Could you check a few things on this model? Use its own coordinates, in mm. A direction names the side the tool comes from. Round coordinates to 2 decimals unless told otherwise and drop trailing zeros. Loops run counter-clockwise (first coordinate to the right, second up) from the corner with the lowest first, then second, coordinate; pieces in that order, holes last. Notation, with made-up numbers: M -26.5,24 L -7.5,24 A22 cw -7.5,48 Z; hole C -10,76.5 d7. An arc over 180 degrees is marked long. Answer in a Markdown table with one row per item.
```python
from build123d import *

# Parameters (mm, degrees)
F1_DEPTH = 436.5625
F2_R     = 5.55625
F3_DEPTH = 50.801
F4_R     = 5.55625
F5_DEPTH = 50.801


with BuildPart() as f1:
    # F0 (on Right) → F1 (new body)
    with BuildSketch(Plane.YZ):
        Polygon((0, 50.8), (0, 0), (50.8, 0), (50.8, 6.35), (6.35, 6.35), (6.35, 50.8), align=None)
    extrude(amount=F1_DEPTH)

    # F2 (on face) → F3 (cut, through all)
    with BuildSketch(Plane.XZ):
        with Locations((25.4, 25.4)):
            Circle(F2_R)
        with BuildLine():
            ThreePointArc((144.4625, 30.1625), (139.7, 25.4), (144.4625, 20.6375))
            Line((144.4625, 20.6375), (160.3375, 20.6375))
            ThreePointArc((160.3375, 20.6375), (165.1, 25.4), (160.3375, 30.1625))
            Line((160.3375, 30.1625), (144.4625, 30.1625))
        make_face()
        with BuildLine():
            ThreePointArc((400.84375, 30.1625), (396.08125, 25.4), (400.84375, 20.6375))
            Line((400.84375, 20.6375), (416.71875, 20.6375))
            ThreePointArc((416.71875, 20.6375), (421.48125, 25.4), (416.71875, 30.1625))
            Line((416.71875, 30.1625), (400.84375, 30.1625))
        make_face()
    extrude(amount=-F3_DEPTH, mode=Mode.SUBTRACT)

    # F4 (on face) → F5 (cut, through all)
    with BuildSketch(Plane(origin=(0, 0, 0), x_dir=(1, 0, 0), z_dir=(0, 0, -1))):
        with Locations((227.80625, -25.4)):
            Circle(F4_R)
        with Locations((177.00625, -25.4)):
            Circle(F4_R)
    extrude(amount=-F5_DEPTH, mode=Mode.SUBTRACT)


solid = f1.part
```
1) I want a section at A-A, the plane y = 25.4. Please give me the cut outline in (x, z), plus the area to 3 significant figures.
Computed:
| item | result |
|---|---|
| outline | M 0,0 L 171.45,0 L 171.45,6.35 L 0,6.35 Z; M 182.56,0 L 222.25,0 L 222.25,6.35 L 182.56,6.35 Z; M 233.36,0 L 436.56,0 L 436.56,6.35 L 233.36,6.35 Z |
| area | 2,630 mm² |
2) I want a section at C-C, the plane x = 25.4. Please give me the cut outline in (y, z).
Computed:
| item | result |
|---|---|
| outline | M 0,0 L 50.8,0 L 50.8,6.35 L 6.35,6.35 L 6.35,19.84 L 0,19.84 Z; M 0,30.96 L 6.35,30.96 L 6.35,50.8 L 0,50.8 Z |
3) Which directions (+Z, -Z, +X, -X, +Y, -Y) give clear straight access to the entire face, cutting with the end or side of a thin tool? Please do faces 1 (the face through (215, 6.35, 28)), 2 (the face through (436.562, 14, 5)).
Computed:
| item | result |
|---|---|
| face 1 | +Z, +X, -X, +Y |
| face 2 | +Z, -Z, +X, +Y, -Y |
4) I want a section at D-D, the plane y = 46. Please give me the cut outline in (x, z), plus the area to 3 significant figures.
Computed:
| item | result |
|---|---|
| outline | M 0,0 L 436.56,0 L 436.56,6.35 L 0,6.35 Z |
| area | 2,770 mm² |
5) I need wall thicknesses on line 1 (X direction, y = 25.4, z = 4.5); line 2 (Z direction, x = 25.4, y = 3.5); line 3 (X direction, y = 1, z = 25). Which ranges of each line are inside material? Lowest first, please.
Computed:
| item | result |
|---|---|
| line 1 | x = 0 to 171.45, 182.56 to 222.25, 233.36 to 436.56 |
| line 2 | z = 0 to 19.84, 30.96 to 50.8 |
| line 3 | x = 0 to 19.86, 30.94 to 139.72, 165.08 to 396.1, 421.46 to 436.56 |
6) I want a section at B-B, the plane z = 25.4. Please give me the cut outline in (x, y), plus the area to 3 significant figures.
Computed:
| item | result |
|---|---|
| outline | M 0,0 L 19.84,0 L 19.84,6.35 L 0,6.35 Z; M 30.96,0 L 139.7,0 L 139.7,6.35 L 30.96,6.35 Z; M 165.1,0 L 396.08,0 L 396.08,6.35 L 165.1,6.35 Z; M 421.48,0 L 436.56,0 L 436.56,6.35 L 421.48,6.35 Z |
| area | 2,380 mm² |
7) Will these pins go through, and if not, where does the flat tip stop? P1, Ø12, axis at x = 226.5, y = 33, coming from the -Z side; P2, Ø13.5, axis at x = 327, y = 20.5, coming from the +Z side; P3, Ø13, axis at x = 25.4, z = 25.4, coming from the +Y side.
Computed:
| item | result |
|---|---|
| P1 | stops at z = 0 |
| P2 | stops at z = 6.35 |
| P3 | stops at y = 6.35 |
8) If we mould it in two halves opening along X, with no side actions, what happens to faces 3 (the face through (172.597, 28.781, 3.131)), 4 (the face through (0, 14, 5)), 5 (the face through (215, 0, 26))? For each: released by +X, released by -X, zero draft, split by the parting line, or undercut.
Computed:
| item | result |
|---|---|
| face 3 | undercut |
| face 4 | released by -X |
| face 5 | zero draft |
